Source: CAD feature listing. Evaluate the final solid. Frame: model axes, mm. A direction names the side the tool comes from. Round coordinates to 2 decimals unless told otherwise and drop trailing zeros. Write each loop counter-clockwise with the first axis right and the second up, starting at its lowest first coordinate (ties: lowest second). Pieces come first, ordered by that corner, then holes. Notation, with made-up numbers: M 80,61.5 L 123,61.5 A10 ccw 123,80.5 Z; hole C 15,-8.5 d3. An arc over 180 degrees is marked long. Answer in a Markdown table with one row per item.
from build123d import *

# Parameters (mm, degrees)
SKETCH_1_R           = 5
EXTRUDE_1_DEPTH      = 4
SKETCH_2_R           = 3.55
EXTRUDE_2_DEPTH      = 0.3
SKETCH_3_R           = 0.6
CUT_EXTRUDE_1_DEPTH  = 9.275868534
SKETCH_4_OUTSIDE_W   = 14.956
SKETCH_4_OUTSIDE_H   = 14.956
SKETCH_4_OUTSIDE_W_2 = 10
SKETCH_4_OUTSIDE_H_2 = 7.1
CUT_EXTRUDE_2_DEPTH  = 9.124038405
FILLET_1_R           = 1.5


with BuildPart() as part:
    # 草图1 → 凸台-拉伸1 (new body)
    with BuildSketch(Plane(origin=(0, 0, 0), x_dir=(1, 0, 0), z_dir=(0, 1, 0))):
        with Locations(Location((0, 0, 0), (0, 0, 270))):
            Circle(SKETCH_1_R)
    extrude(amount=EXTRUDE_1_DEPTH)

    # 草图2 → 凸台-拉伸2 (add)
    with BuildSketch(Plane(origin=(0, 4, 0), x_dir=(1, 0, 0), z_dir=(0, 1, 0))):
        with Locations(Location((0, 0, 0), (0, 0, 270))):
            Circle(SKETCH_2_R)
    extrude(amount=EXTRUDE_2_DEPTH)

    # 草图3 → 切除-拉伸1 (cut, through all)
    with BuildSketch(Plane(origin=(0, 4.3, 0), x_dir=(1, 0, 0), z_dir=(0, 1, 0))):
        with Locations(Location((0, 0, 0), (0, 0, 270))):
            Circle(SKETCH_3_R)
    extrude(amount=-CUT_EXTRUDE_1_DEPTH, mode=Mode.SUBTRACT)

    # 草图4 outside → 切除-拉伸2 (cut, through all)
    with BuildSketch(Plane(origin=(0, 4, 0), x_dir=(1, 0, 0), z_dir=(0, 1, 0))):
        Rectangle(SKETCH_4_OUTSIDE_W, SKETCH_4_OUTSIDE_H)
        Rectangle(SKETCH_4_OUTSIDE_W_2, SKETCH_4_OUTSIDE_H_2, mode=Mode.SUBTRACT)
    extrude(amount=-CUT_EXTRUDE_2_DEPTH, mode=Mode.SUBTRACT)

    # 圆角1
    # the kernel refuses this fillet: 1.5 mm, written as the material it takes off along each edge
    with BuildSketch(Plane(origin=(0, 0, 0), x_dir=(-0.03098871975283517, 0, 0.9995197342964671), z_dir=(0.9995197342964671, 0, 0.03098871975283517))) as fillet_1_piece_1:
        with BuildLine():
            CenterArc((5 - FILLET_1_R, -FILLET_1_R), FILLET_1_R, 0, 90)
            Line((5 - FILLET_1_R, 0), (5, 0))
            Line((5, 0), (5, -FILLET_1_R))
        make_face()
    revolve(axis=Axis((0, 0, 0), (0, -1, 0)), revolution_arc=176.4483857, mode=Mode.SUBTRACT)
    with BuildSketch(Plane(origin=(-7.271008378, 0, -3.55), x_dir=(0, 1, 0), z_dir=(1, 0, 0)), Plane(origin=(7.271008378, 0, 3.55), x_dir=(0, 1, 0), z_dir=(-1, 0, 0))) as fillet_1_piece_2:
        with BuildLine():
            CenterArc((FILLET_1_R, FILLET_1_R), FILLET_1_R, 180, 90)
            Line((0, FILLET_1_R), (0, 0))
            Line((0, 0), (FILLET_1_R, 0))
        make_face()
    extrude(amount=14.542016757, mode=Mode.SUBTRACT)
    with BuildSketch(Plane(origin=(0, 0, 0), x_dir=(0.030988719752834452, 0, 0.9995197342964671), z_dir=(-0.9995197342964671, 0, 0.030988719752834452))) as fillet_1_piece_3:
        with BuildLine():
            CenterArc((5 - FILLET_1_R, FILLET_1_R), FILLET_1_R, 270, 90)
            Line((5 - FILLET_1_R, 0), (5, 0))
            Line((5, 0), (5, FILLET_1_R))
        make_face()
    revolve(axis=Axis((0, 0, 0), (0, 1, 0)), revolution_arc=176.4483857, mode=Mode.SUBTRACT)


solid = part.part
Q1. Section A-A (z = 0). Return loops of the section in (x, y).
Solutions:
| item | result |
|---|---|
| outline | M -5,1.5 A1.5 ccw -3.5,0 L -0.6,0 L -0.6,4.3 L -3.55,4.3 L -3.55,4 L -5,4 Z; M 0.6,0 L 3.5,0 A1.5 ccw 5,1.5 L 5,4 L 3.55,4 L 3.55,4.3 L 0.6,4.3 Z |
Q2. Pull-direction query (Z, two-part tool) for faces 4 (the cylindrical face through (0.506, 2.18, 0.323)), 5 (the flat face through (4, 4, 0)), 6 (the flat face through (0, 3, 3.55)); classes: pulls with the +Z half, pulls with the -Z half, needs draft (parallel to the pull), parting line crosses it, or undercut.
Solutions:
| item | result |
|---|---|
| face 4 | undercut |
| face 5 | needs draft |
| face 6 | pulls with the +Z half |
Q3. Material intervals for probe 1 along X at (y, z) = (1.5, 0); probe 2 along Z at (x, y) = (0.5, 3.75); probe 3 along X at (y, z) = (2.65, 0.5), sorted ascending.
Solutions:
| item | result |
|---|---|
| probe 1 | x = -5 to -0.6, 0.6 to 5 |
| probe 2 | z = -3.55 to -0.33, 0.33 to 3.55 |
| probe 3 | x = -4.97 to -0.33, 0.33 to 4.97 |
Q4. Section D-D (x = -1). Return loops of the section in (y, z), and give its area (3 significant figures).
Solutions:
| item | result |
|---|---|
| outline | M 0,-2.05 A1.5 ccw 1.5,-3.55 L 4,-3.55 L 4,-3.41 L 4.3,-3.41 L 4.3,3.41 L 4,3.41 L 4,3.55 L 1.5,3.55 A1.5 ccw 0,2.05 Z |
| area | 29.5 mm2 |
Q5. Contact query for flat-ended pins moving along their axis: pin 1 Ø1.5 at (y, z) = (1.5, -1.5) entering from +X; pin 2 Ø2 at (y, z) = (2.5, -1.5) entering from -X. Output: stop coordinate, or through.
Solutions:
| item | result |
|---|---|
| pin 1 | stops at x = 4.94 |
| pin 2 | stops at x = -4.97 |
Q6. Section C-C (x = 1.5). Return loops of the section in (y, z).
Solutions:
| item | result |
|---|---|
| outline | M 0,-2.05 A1.5 ccw 1.5,-3.55 L 4,-3.55 L 4,-3.22 L 4.3,-3.22 L 4.3,3.22 L 4,3.22 L 4,3.55 L 1.5,3.55 A1.5 ccw 0,2.05 Z |
Q7. Section B-B (y = 1.7). Return loops of the section in (x, z), and give its area (3 significant figures).
Solutions:
| item | result |
|---|---|
| outline | M -3.52,-3.55 L 3.52,-3.55 A5 ccw 3.52,3.55 L -3.52,3.55 A5 ccw Z; hole C 0,0 d1.2 |
| area | 63.3 mm2 |
Q8. Access query for faces 1 (the flat face through (-4, 4, 0)), 2 (the cylindrical face through (-1.36, 4.15, 3.28)), 3 (the flat face through (0, 3, -3.55)). Directions: +Z, -Z, +X, -X, +Y, -Y. A direction counts if a zero-diameter tool reaches every point of the face in a straight line with its end or side. Return the directions, or none.
Solutions:
| item | result |
|---|---|
| face 1 | -X, +Y |
| face 2 | +Y |
| face 3 | -Z, +X, -X, +Y, -Y |
